from build123d import *

# Parameters (mm, degrees)
EXTRUDE_THIN1_0_090_DEPTH       = 139.7
BE_00_FRONT_BEARING_PLATE_DEPTH = 9.525
SKETCH10_R                      = 2.7813
SKETCH10_R_2                    = 11.1125
SKETCH10_R_3                    = 28.575
CE_00_FRONT_HOLES_DEPTH         = 25.4
SKETCH11_R                      = 6.35
CE_00_UPPOER_HOLES_DEPTH        = 25.4
SKETCH12_R                      = 6.5532
CE_00_LOWER_HOLES_DEPTH         = 12.7
BE_00_START                     = -127
BE_00_SIDE_PANEL_DEPTH          = 3.175


with BuildPart() as part:
    # Sketch9 → Extrude-Thin1 0.090 (new, symmetric)
    with BuildSketch(Plane.XY):
        Polygon((-6.010227149, -332.418181598), (9.55556721, -304.745658294), (384.039485631, -120.64961833), (425.625062176, -27.95010472), (2.683531334, 161.784088268), (4.161010967, 201.456785856), (6.445427335, 201.371710254), (5.025301148, 163.239044684), (428.646476704, -26.800041136), (385.787807265, -122.337439943), (11.200381601, -306.484363998), (-4.017805471, -333.538918792), align=None)
    extrude(amount=EXTRUDE_THIN1_0_090_DEPTH, both=True)

    # Sketch13 → BE-00 Front Bearing Plate (add)
    with BuildSketch(Plane(origin=(366.842913711, -164.56800553, 0), x_dir=(0, 0, -1), z_dir=(0.9123967874925901, -0.40930685576129966, 0))):
        with BuildLine():
            Line((-127, 145.534670176), (127, 145.534670176))
            ThreePointArc((127, 145.534670176), (135.980256121, 141.814926297), (139.7, 132.834670176))
            Line((139.7, 132.834670176), (139.7, 62.984670176))
            ThreePointArc((139.7, 62.984670176), (135.980256121, 54.004414055), (127, 50.284670176))
            Line((127, 50.284670176), (-127, 50.284670176))
            ThreePointArc((-127, 50.284670176), (-135.980256121, 54.004414055), (-139.7, 62.984670176))
            Line((-139.7, 62.984670176), (-139.7, 132.834670176))
            ThreePointArc((-139.7, 132.834670176), (-135.980256121, 141.814926297), (-127, 145.534670176))
        make_face()
    extrude(amount=BE_00_FRONT_BEARING_PLATE_DEPTH)

    # Sketch10 → CE-00 Front Holes (cut)
    with BuildSketch(Plane(origin=(-463.262854861, -2038.249879483, 0), x_dir=(0, 0, -1), z_dir=(-0.9123967874925901, 0.40930685576129966, 0))):
        with Locations(Location((-118.013029727, -2185.318974837, 0), (0, 0, 270))):
            Circle(SKETCH10_R)
        with Locations(Location((0, -2147.218974837, 0), (0, 0, 270))):
            Circle(SKETCH10_R_2)
        with Locations(Location((57.15, -2147.218974837, 0), (0, 0, 270))):
            Circle(SKETCH10_R_3)
        with Locations(Location((114.3, -2109.118974837, 0), (0, 0, 270))):
            Circle(SKETCH10_R)
        with Locations(Location((118.013029727, -2185.318974837, 0), (0, 0, 270))):
            Circle(SKETCH10_R)
        with Locations(Location((0, -2109.118974837, 0), (0, 0, 270))):
            Circle(SKETCH10_R)
        with Locations(Location((0, -2185.318974837, 0), (0, 0, 270))):
            Circle(SKETCH10_R)
        with Locations(Location((-114.3, -2109.118974837, 0), (0, 0, 270))):
            Circle(SKETCH10_R)
        with Locations(Location((-57.15, -2147.218974837, 0), (0, 0, 270))):
            Circle(SKETCH10_R_3)
    extrude(amount=CE_00_FRONT_HOLES_DEPTH, mode=Mode.SUBTRACT)

    # Sketch11 → CE-00 Uppoer Holes (cut)
    with BuildSketch(Plane(origin=(-26.304972354, -678.029043238, 0), x_dir=(0, 0, -1), z_dir=(-0.9993072475406022, 0.037215924183416293, 0))):
        with Locations(Location((-117.475, -860.185852954, 0), (0, 0, 270))):
            Circle(SKETCH11_R)
        with Locations(Location((0, -860.185852954, 0), (0, 0, 270))):
            Circle(SKETCH11_R)
        with Locations(Location((117.475, -860.185852954, 0), (0, 0, 270))):
            Circle(SKETCH11_R)
    extrude(amount=CE_00_UPPOER_HOLES_DEPTH, mode=Mode.SUBTRACT)

    # Sketch12 → CE-00 Lower Holes (cut, symmetric)
    with BuildSketch(Plane(origin=(139.468979542, -78.451300992, 0), x_dir=(0, 0, -1), z_dir=(0.8715755371243086, -0.49026123963298696, 0))):
        with Locations(Location((101.6, -280.036485408, 0), (0, 0, 90))):
            Circle(SKETCH12_R)
        with Locations(Location((50.8, -280.036485408, 0), (0, 0, 90))):
            Circle(SKETCH12_R)
        with Locations(Location((-50.8, -280.036485408, 0), (0, 0, 90))):
            Circle(SKETCH12_R)
        with Locations(Location((-101.6, -280.036485408, 0), (0, 0, 90))):
            Circle(SKETCH12_R)
        with BuildLine():
            Line((-19.05, -253.366485408), (19.05, -253.366485408))
            ThreePointArc((19.05, -253.366485408), (23.540128061, -255.226357347), (25.4, -259.716485408))
            Line((25.4, -259.716485408), (25.4, -304.513722271))
            Line((25.4, -304.513722271), (-25.4, -304.513722271))
            Line((-25.4, -304.513722271), (-25.4, -259.716485408))
            ThreePointArc((-25.4, -259.716485408), (-23.540128061, -255.226357347), (-19.05, -253.366485408))
        make_face()
    extrude(amount=CE_00_LOWER_HOLES_DEPTH, both=True, mode=Mode.SUBTRACT)

    # Sketch14 → BE-00 Side Panel (add)
    with BuildSketch(Plane.XY.offset(BE_00_START)):
        Polygon((2.683531334, 161.784088268), (425.625062176, -27.95010472), (384.039485631, -120.64961833), (9.55556721, -304.745658294), align=None)
    be_00_side_panel = extrude(amount=BE_00_SIDE_PANEL_DEPTH)

    # MI-00 Side Panel: BE-00 Side Panel across plane
    add(be_00_side_panel.mirror(Plane.XY))


solid = part.part
Geometry: final body of the model. Coordinates: model frame, mm. A direction names the side the tool comes from. Give positions to 0.01 mm unless a question says otherwise; leave off trailing zeros. Write each loop counter-clockwise with the first axis right and the second up, starting at its lowest first coordinate (ties: lowest second). Pieces come first, ordered by that corner, then holes.
(1) Cut plane C-C, the plane y = 63.5. Return loops of the section in (x, z) (3 decimals).
(2) Cut plane B-B, the plane x = 307. Return loops of the section in (y, z) (3 decimals), then the cut area to 3 significant figures.
(3) First-contact query: P1, Ø10, axis at x = 309, z = -7.5, coming from the -Y side; P2, Ø10, axis at y = 120, z = -2, coming from the -X side; P3, Ø3, axis at y = -53, z = 83.5, coming from the -X side. Flat tips, straight axial feed; report the tip coordinate or a pass-through.
(4) Cut plane D-D, the plane z = 71. Return loops of the section in (x, y), then the cut area to 3 significant figures.
(5) Ray query, line 1 (Z direction, x = 185, y = -56.5) (3 decimals); line 2 (Y direction, x = 300, z = 97); line 3 (Y direction, x = 320, z = -35). Return the intervals inside material, ascending.
(6) Access query for faces 3 (the flat face through (404.54, -74.95, -133.26)), 4 (the cylindrical face through (4.26, -316.524, 52.768)), 5 (the flat face through (170, -68, 123.825)), 6 (the flat face through (1.66, -318.78, -81.75)), 7 (the flat face through (6.06, 191.05, 1.96)). Directions: +Z, -Z, +X, -X, +Y, -Y. A direction counts if a zero-diameter tool reaches every point of the face in a straight line with its end or side. Return the directions, or none.
(7) Mould query, pull axis Z, two halves, no side actions, for faces 1 (the cylindrical face through (4.71, 185.01, -122.83)), 2 (the flat face through (194.176, -213.986, 133.439)). Classes: released by +Z, released by -Z, zero draft, split by the parting line, or undercut.
(8) Cut plane A-A, the plane z = -79. Return loops of the section in (x, y), then the cut area to 3 significant figures.
Values follow:
1. outline: (4.131, -127) - (221.771, -127) - (221.771, -139.7) - (227.356, -139.7) - (227.356, 139.7) - (221.771, 139.7) - (221.771, 127) - (4.131, 127) - (4.131, 123.825) - (221.771, 123.825) - (221.771, -123.825) - (4.131, -123.825) - close
2. outline: (-161.069, -139.7) - (-158.522, -139.7) - (-158.522, -127) - (25.266, -127) - (25.266, -139.7) - (27.771, -139.7) - (27.771, 139.7) - (25.266, 139.7) - (25.266, 127) - (-158.522, 127) - (-158.522, 139.7) - (-161.069, 139.7) - close; hole (-158.522, -123.825) - (25.266, -123.825) - (25.266, 123.825) - (-158.522, 123.825) - close
2. area: 2,580 mm2
3. P1: stops at y = -162.54
3. P2: stops at x = 84.68
3. P3: stops at x = 413.71
4. outline: (-6.01, -332.42) - (-4.02, -333.54) - (11.2, -306.48) - (385.79, -122.34) - (387.42, -118.69) - (396.12, -122.59) - (405.38, -101.94) - (394.6, -97.1) - (384.04, -120.65) - (9.56, -304.75) - close; (2.68, 161.78) - (425.63, -27.95) - (415.06, -51.5) - (425.84, -56.33) - (435.1, -35.68) - (426.41, -31.78) - (428.65, -26.8) - (5.03, 163.24) - (6.45, 201.37) - (4.16, 201.46) - close
4. area: 2,730 mm2
5. line 1: z = -127 to -123.825, 123.825 to 127
5. line 2: y = -164.51 to -161.96, 28.41 to 30.91
5. line 3: y = -154.68 to -152.13, 19.43 to 21.94
6. face 3: -Z, -X
6. face 4: none
6. face 5: -X
6. face 6: +Z, -Z, -X
6. face 7: +Z, -Z, +X
7. face 1: undercut
7. face 2: zero draft
8. outline: (-6.01, -332.42) - (-4.02, -333.54) - (11.2, -306.48) - (385.79, -122.34) - (387.42, -118.69) - (396.12, -122.59) - (408.07, -95.94) - (397.29, -91.1) - (384.04, -120.65) - (9.56, -304.75) - close; (2.68, 161.78) - (425.63, -27.95) - (412.37, -57.5) - (423.15, -62.33) - (435.1, -35.68) - (426.41, -31.78) - (428.65, -26.8) - (5.03, 163.24) - (6.45, 201.37) - (4.16, 201.46) - close
8. area: 2,880 mm2
